```python
from build123d import *

# Parameters (mm, degrees)
F1_DEPTH = 12.7
F0_W     = 76.2
F0_H     = 101.6
F2_DEPTH = 63.5
F4_D     = 76.2


with BuildPart() as f1:
    # F0 (on Front) → F1 (new body, symmetric)
    with BuildSketch(Plane.XZ):
        Polygon((146.07237, -15.042048), (-31.72763, 86.557952), (-31.72763, -15.042048), align=None)
    extrude(amount=F1_DEPTH, both=True)

    # F0 (on Front) → F2 (join, symmetric)
    with BuildSketch(Plane.XZ):
        with Locations((-69.82763, 35.757952)):
            Rectangle(F0_W, F0_H)
        Polygon((146.07237, -65.842048), (146.07237, -15.042048), (-31.72763, -15.042048), (-107.92763, -15.042048), (-107.92763, -65.842048), (19.07237, -65.842048), (-4.595719, -42.173959), (118.940459, -42.173959), (95.27237, -65.842048), align=None)
    extrude(amount=F2_DEPTH, both=True)

    # F4 (through all)
    with Locations(Plane.XY.offset(86.557952)):
        with Locations((-107.92763, 0)):
            Hole(F4_D / 2)


solid = f1.part
```
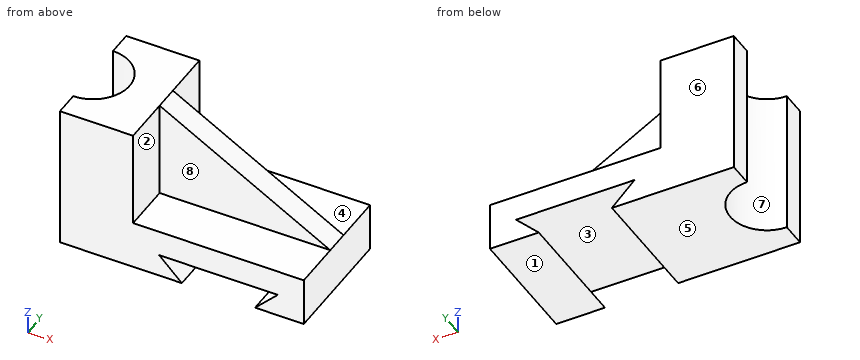
For this review, take the finished solid that the model builds, in its own axes (mm). Face numbers are marked on the shaded views. A direction names the side the tool comes from. Coordinates: 2 decimals unless noted, no trailing zeros. Write each loop counter-clockwise with the first axis right and the second up, starting at its lowest first coordinate (ties: lowest second). Pieces come first, ordered by that corner, then holes. Notation, with made-up numbers: (49.25, 59.25) -> (80.25, 59.25) arc R25 ccw to (80.25, 71.25) -> close; hole circle Ø4 at (-23.75, 7.5). An arc over 180 degrees is marked (long way). Put each result on its own line as item: value.
Q1. Wall thickness on L1, parallel to Z at x = 28.5, y = 26; L2, parallel to Z at x = -11.5, y = -18.5; L3, parallel to Z at x = 113.5, y = 56.5: over which ranges is each line inside the solid? List them lowest first.
From the geometry:
L1: z = -42.17 to -15.04
L2: z = -65.84 to -15.04
L3: z = -65.84 to -47.61, -42.17 to -15.04
Q2. Take a section at C-C, the plane x = -85.5. State the section outline as (y, z) points, then the cut area to 3 significant figures.
From the geometry:
outline: (-63.5, -65.84) -> (-30.8, -65.84) -> (-30.8, 86.56) -> (-63.5, 86.56) -> close; (30.8, -65.84) -> (63.5, -65.84) -> (63.5, 86.56) -> (30.8, 86.56) -> close
area: 9,970 mm2
Q3. Take a section at B-B, the plane z = -37.5. State the section outline as (x, y) points, then the cut area to 3 significant figures.
From the geometry:
outline: (-107.93, -63.5) -> (146.07, -63.5) -> (146.07, 63.5) -> (-107.93, 63.5) -> (-107.93, 38.1) arc R38.1 cw to (-107.93, -38.1) -> close
area: 30,000 mm2
Q4. Clearance check with flat-ended pins moving along their axes: pin 1 Ø15 at (x, y) = (46.5, 44.5) entering from +Z; pin 2 Ø3 at (y, z) = (-10, 22.5) entering from +X; pin 3 Ø4 at (x, z) = (27, -13) entering from -Y. State where each tip first meets the part, or that it passes through.
From the geometry:
pin 1: stops at z = -15.04
pin 2: stops at x = 83
pin 3: stops at y = -12.7
Q5. Tool access review of the marked faces 1, 2, 3 and 4: name each direction out of +Z, -Z, +X, -X, +Y, -Y from which nothing blocks a thin tool from reaching the whole face with its end or side.
From the geometry:
face 1: -Z, +X, -X, +Y, -Y
face 2: +Z, +X, -Y
face 3: +Y, -Y
face 4: +Z, +X, +Y
Q6. Take a section at D-D, the plane x = -13.5. State the section outline as (y, z) points, then the cut area to 3 significant figures.
From the geometry:
outline: (-63.5, -65.84) -> (63.5, -65.84) -> (63.5, -15.04) -> (12.7, -15.04) -> (12.7, 76.14) -> (-12.7, 76.14) -> (-12.7, -15.04) -> (-63.5, -15.04) -> close
area: 8,770 mm2
Q7. The part is to be moulded in two halves that separate along Y. For the marked faces 5, 6, 7 and 8, say which applies: +Y half, -Y half, draft (parallel to the pull), parting line (faces both ways), or undercut.
From the geometry:
face 5: draft
face 6: +Y half
face 7: undercut
face 8: -Y half
Q8. Take a section at A-A, the plane y = 0. State the section outline as (x, z) points.
From the geometry:
outline: (-69.83, -65.84) -> (19.07, -65.84) -> (-4.6, -42.17) -> (118.94, -42.17) -> (95.27, -65.84) -> (146.07, -65.84) -> (146.07, -15.04) -> (-31.73, 86.56) -> (-69.83, 86.56) -> close
